Read the model definition and answer for the solid it produces. Units are mm, in the model's axes. Face numbers are marked on the shaded views. A direction names the side the tool comes from. Give positions to 0.01 mm unless a question says otherwise; leave off trailing zeros. Order: outer loops, then holes, each group sorted by start corner. A loop starts at its lowest first (then second) coordinate and runs counter-clockwise, first axis right, second up. Notation, with made-up numbers: (30, -35.5) - (64, -35.5) arc R22 ccw to (64, -5.5) - close; hole circle Ø7 at (-27, 0). An arc over 180 degrees is marked (long way). Return JSON: item names as keys, results as strings.
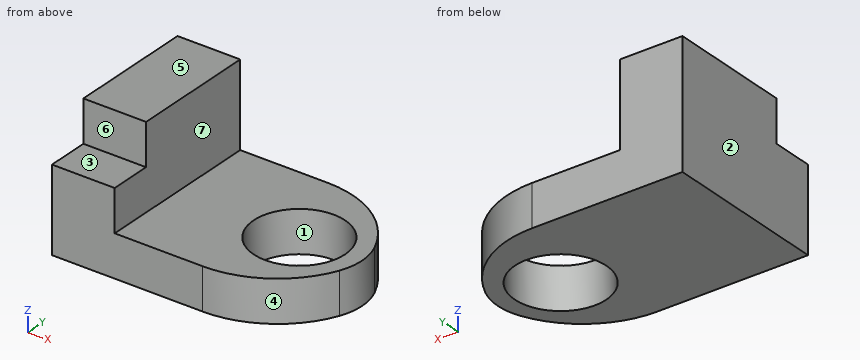
```python
from build123d import *

# Parameters (mm, degrees)
F1_DEPTH = 12.7
F2_W     = 19.05
F2_H     = 50.8
F3_DEPTH = 25.4
F4_W     = 19.05
F4_H     = 12.7
F5_DEPTH = 12.7
F6_R     = 13.8806094442
F7_DEPTH = 12.7
F8_R     = 17.78


with BuildPart() as f1:
    # F0 (on Top) → F1 (new body)
    with BuildSketch(Plane.XY):
        with BuildLine():
            ThreePointArc((37.6736852981, 0), (27.2947553987, 18.1994845304), (7.62, 25.4))
            Line((7.62, 25.4), (-38.1, 25.4))
            Line((-38.1, 25.4), (-38.1, -25.4))
            Line((-38.1, -25.4), (7.62, -25.4))
            ThreePointArc((7.62, -25.4), (27.2947553987, -18.1994845304), (37.6736852981, 0))
        make_face()
    extrude(amount=F1_DEPTH)

    # F2 (on face) → F3 (join)
    with BuildSketch(Plane.XY.offset(12.7)):
        with Locations((-28.575, 0)):
            Rectangle(F2_W, F2_H)
    extrude(amount=F3_DEPTH)

    # F4 (on face) → F5 (cut)
    with BuildSketch(Plane.XY.offset(38.1)):
        with Locations((-28.575, -19.05)):
            Rectangle(F4_W, F4_H)
    extrude(amount=-F5_DEPTH, mode=Mode.SUBTRACT)

    # F6 (on face) → F7 (cut)
    with BuildSketch(Plane.XY.offset(12.7)):
        with Locations((18.0154964328, 0)):
            Circle(F6_R)
    extrude(amount=-F7_DEPTH, mode=Mode.SUBTRACT)

    # F8
    f8_edges = [f1.edges().sort_by_distance(p)[0] for p in [
        (37.673685, 0, 6.35),
    ]]
    fillet(f8_edges, radius=F8_R)


solid = f1.part
```
Q1. Consider L1, parallel to Z at x = -2.5, y = -13; L2, parallel to X at y = -3.5, z = 3; L3, parallel to X at y = 1, z = 18. Determine where each line is inside the solid, lowest interval first.
Values:
{"L1": "z = 0 to 12.7", "L2": "x = -38.1 to 4.58, 31.45 to 36.69", "L3": "x = -38.1 to -19.05"}
Q2. A cutting plane is placed at B-B (x = 1.5). Write down the section's boundary in (y, z).
Values:
{"outline": "(-25.4, 0) - (25.4, 0) - (25.4, 12.7) - (-25.4, 12.7) - close"}
Q3. A cutting plane is placed at D-D (y = 15.5). Write down the section's boundary in (x, z).
Values:
{"outline": "(-38.1, 0) - (30.1, 0) - (30.1, 12.7) - (-19.05, 12.7) - (-19.05, 38.1) - (-38.1, 38.1) - close"}
Q4. For the marked faces 5, 6 and 7, determine the directions among +Z, -Z, +X, -X, +Y, -Y from which every point of the face is accessible in a straight line to the end or side of a thin tool.
Values:
{"face 5": "+Z, +X, -X, +Y, -Y", "face 6": "+Z, +X, -X, -Y", "face 7": "+Z, +X, +Y, -Y"}
Q5. A cutting plane is placed at A-A (y = 8). Write down the section's boundary in (x, z), and give its area (3 significant figures).
Values:
{"outline": "(-38.1, 0) - (6.67, 0) - (6.67, 12.7) - (-19.05, 12.7) - (-19.05, 38.1) - (-38.1, 38.1) - close; (29.36, 0) - (35.15, 0) - (35.15, 12.7) - (29.36, 12.7) - close", "area": "1,130 mm²"}
Q6. A cutting plane is placed at C-C (y = -15). Write down the section's boundary in (x, z), and give its area (3 significant figures).
Values:
{"outline": "(-38.1, 0) - (30.55, 0) - (30.55, 12.7) - (-19.05, 12.7) - (-19.05, 25.4) - (-38.1, 25.4) - close", "area": "1,110 mm²"}
Q7. Determine the mould class of the marked faces 1, 2, 3 and 4 for opening direction X: released by +X, released by -X, zero draft, split by the parting line, or undercut.
Values:
{"face 1": "undercut", "face 2": "released by -X", "face 3": "zero draft", "face 4": "released by +X"}
Q8. Given pin 1 (2 mm diameter, centred on x = -26.5, y = -7, fed in from -Z); pin 2 (6.5 mm diameter, centred on x = -33, z = 32, fed in from -Y); pin 3 (7.5 mm diameter, centred on y = 8, z = 25.5, fed in from +X); pin 4 (3 mm diameter, centred on x = 9, y = -14.5, fed in from +Z), each flat-ended and moving along its own axis, determine where each tip first touches the part or whether it passes through.
Values:
{"pin 1": "stops at z = 0", "pin 2": "stops at y = -12.7", "pin 3": "stops at x = -19.05", "pin 4": "stops at z = 12.7"}
